Here's how the part is built. I have some questions about the finished solid (model axes, mm). Face numbers are marked on the shaded views. A direction names the side the tool comes from. Give positions to 0.01 mm unless a question says otherwise; leave off trailing zeros. Loops run counter-clockwise (first coordinate to the right, second up) from the corner with the lowest first, then second, coordinate; pieces in that order, holes last. Notation, with made-up numbers: (22, 53.25) -> (31, 53.25) arc R17 cw to (31, 63.25) -> close; hole circle Ø3 at (73, 34.5). An arc over 180 degrees is marked (long way). Answer in a Markdown table with one row per item. Add a question column.
Item 1: Which directions (+Z, -Z, +X, -X, +Y, -Y) give clear straight access to the entire face, cutting with the end or side of a thin tool? Please do the marked faces 1, 2 and 3.
Item 2: If we section it at B-B (y = 0): Write out the boundary of the cut face in (x, z), then the cut area to 3 significant figures.
Item 3: If we section it at C-C (z = 34): Write out the boundary of the cut face in (x, y).
Item 4: If we section it at A-A (x = 0): Write out the boundary of the cut face in (y, z), then the cut area to 3 significant figures.
Item 5: For P1, Ø3, axis at y = 39.5, z = 26.5, coming from the -X side; P2, Ø2, axis at y = -16.5, z = 28, coming from the +X side; P3, Ø5, axis at y = -10, z = 36, coming from the -X side; P4, Ø16, axis at x = -5, y = -30, coming from the -Z side, each with a flat end and sliding along its axis, tell me the tip position at first contact or that it passes through.
Item 6: If I drill on line 1 (Y direction, x = 0, z = 27); line 2 (Z direction, x = 38, y = -38), over which ranges is the centre line in solid material (lowest first)?
Item 7: If we section it at D-D (z = 13.5): Write out the boundary of the cut face in (x, y).
Item 8: We'd pull the mould along X, two halves only. Please class the marked faces 4, 5 and 6: released by +X, released by -X, zero draft, split by the parting line, or undercut.
```python
from build123d import *

# Parameters (mm, degrees)
F0_R     = 50.8
F0_R_2   = 44.45
F1_DEPTH = 31.75
F3_DEPTH = 6.35
F4_R     = 44.45
F5_DEPTH = 25.4


with BuildPart() as f1:
    # F0 (on Top) → F1 (new body)
    with BuildSketch(Plane.XY):
        Circle(F0_R)
        Circle(F0_R_2, mode=Mode.SUBTRACT)
    extrude(amount=F1_DEPTH)

    # F2 (on face) → F3 (join)
    with BuildSketch(Plane.XY.offset(31.75)):
        with BuildLine():
            Line((-50.613235, -1.072882), (-50.613235, -26.540967))
            ThreePointArc((-50.613235, -26.540967), (0, -57.15), (50.613235, -26.540967))
            Line((50.613235, -26.540967), (50.613235, 26.540967))
            ThreePointArc((50.613235, 26.540967), (0, 57.15), (-50.613235, 26.540967))
            Line((-50.613235, 26.540967), (-50.613235, -1.072882))
        make_face()
    extrude(amount=F3_DEPTH)

    # F4 (on face) → F5 (cut)
    with BuildSketch(Plane(origin=(0, 0, 31.75), x_dir=(1, 0, 0), z_dir=(0, 0, -1))):
        Circle(F4_R)
    extrude(amount=-F5_DEPTH, mode=Mode.SUBTRACT)


solid = f1.part
```
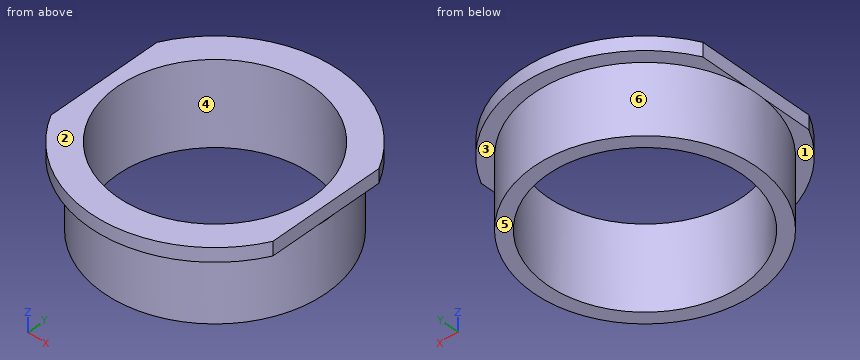
Recorded:
| question | item | result |
|---|---|---|
| 1 | face 1 | -Z, -Y |
| 1 | face 2 | +Z, +X, -X, +Y, -Y |
| 1 | face 3 | -Z, +Y |
| 2 | outline | (-50.8, 0) -> (-44.45, 0) -> (-44.45, 38.1) -> (-50.61, 38.1) -> (-50.61, 31.75) -> (-50.8, 31.75) -> close; (44.45, 0) -> (50.8, 0) -> (50.8, 31.75) -> (50.61, 31.75) -> (50.61, 38.1) -> (44.45, 38.1) -> close |
| 2 | area | 481 mm^2 |
| 3 | outline | (-50.61, -26.54) arc R57.15 ccw to (50.61, -26.54) -> (50.61, 26.54) arc R57.15 ccw to (-50.61, 26.54) -> close; hole circle Ø88.9 at (0, 0) |
| 4 | outline | (-57.15, 31.75) -> (-50.8, 31.75) -> (-50.8, 0) -> (-44.45, 0) -> (-44.45, 38.1) -> (-57.15, 38.1) -> close; (44.45, 0) -> (50.8, 0) -> (50.8, 31.75) -> (57.15, 31.75) -> (57.15, 38.1) -> (44.45, 38.1) -> close |
| 4 | area | 565 mm^2 |
| 5 | P1 | stops at x = -33.71 |
| 5 | P2 | stops at x = 48.38 |
| 5 | P3 | stops at x = -50.61 |
| 5 | P4 | passes through |
| 6 | line 1 | y = -50.8 to -44.45, 44.45 to 50.8 |
| 6 | line 2 | z = 31.75 to 38.1 |
| 7 | outline | circle Ø101.6 at (0, 0); hole circle Ø88.9 at (0, 0) |
| 8 | face 4 | undercut |
| 8 | face 5 | zero draft |
| 8 | face 6 | split by the parting line |
